Read the model definition and answer for the solid it produces. Units are mm, in the model's axes. Face numbers are marked on the shaded views. A direction names the side the tool comes from. Give positions to 0.01 mm unless a question says otherwise; leave off trailing zeros. Write each loop counter-clockwise with the first axis right and the second up, starting at its lowest first coordinate (ties: lowest second). Pieces come first, ordered by that corner, then holes. Notation, with made-up numbers: (-30.75, 18) - (-22.75, 18) arc R20 cw to (-22.75, 32) - close; hole circle Ø3 at (2, -23.75). An arc over 180 degrees is marked (long way). Answer as CSV lines item,"result".
```python
from build123d import *

# Parameters (mm, degrees)
SKICA1_W                 = 55
SKICA1_H                 = 25
P_IDAT_VYSUNUT_M1_DEPTH  = 5
ODEBRAT_VYSUNUT_M1_DEPTH = 10
SKICA3_W                 = 15
SKICA3_H                 = 25
ODEBRAT_VYSUNUT_M2_DEPTH = 2.5
M4_D_RA_S_V_L_4_DEPTH    = 2.5


# Read off the part's stored shape, not the designer's step: M4 díra s vůlí4
with BuildPart() as part:
    # Skica1 → Přidat vysunutím1 (new body)
    with BuildSketch(Plane.XY):
        Rectangle(SKICA1_W, SKICA1_H)
    extrude(amount=P_IDAT_VYSUNUT_M1_DEPTH)

    # Skica2 → Odebrat vysunutím1 (cut)
    with BuildSketch(Plane.XY.offset(5)):
        with BuildLine():
            Line((-12.5, 3.5), (-8.1, 3.5))
            ThreePointArc((-8.1, 3.5), (-7.936021317, 2.6864759), (-7.469693846, 2))
            Line((-7.469693846, 2), (-4.530306154, 2))
            ThreePointArc((-4.530306154, 2), (-4.063978683, 2.6864759), (-3.9, 3.5))
            Line((-3.9, 3.5), (-2.1, 3.5))
            ThreePointArc((-2.1, 3.5), (-1.936021317, 2.6864759), (-1.469693846, 2))
            Line((-1.469693846, 2), (1.469693846, 2))
            ThreePointArc((1.469693846, 2), (1.936021317, 2.6864759), (2.1, 3.5))
            Line((2.1, 3.5), (3.9, 3.5))
            ThreePointArc((3.9, 3.5), (4.063978683, 2.6864759), (4.530306154, 2))
            Line((4.530306154, 2), (7.469693846, 2))
            ThreePointArc((7.469693846, 2), (7.936021317, 2.6864759), (8.1, 3.5))
            Line((8.1, 3.5), (12.5, 3.5))
            Line((12.5, 3.5), (12.5, 12.5))
            Line((12.5, 12.5), (-12.5, 12.5))
            Line((-12.5, 12.5), (-12.5, 3.5))
        make_face()
    extrude(amount=-ODEBRAT_VYSUNUT_M1_DEPTH, mode=Mode.SUBTRACT)

    # Skica3 → Odebrat vysunutím2 (cut)
    with BuildSketch(Plane.XY.offset(5)):
        with Locations((-20, 0)):
            Rectangle(SKICA3_W, SKICA3_H)
        with Locations((20, 0)):
            Rectangle(SKICA3_W, SKICA3_H)
    extrude(amount=-ODEBRAT_VYSUNUT_M2_DEPTH, mode=Mode.SUBTRACT)

    # M4 díra s vůlí4 outline → M4 díra s vůlí4 (cut)
    with BuildSketch(Plane.XY):
        with BuildLine():
            Line((-20.25, 12.5), (-24.75, 12.5))
            Line((-24.75, 12.5), (-24.75, -7.75))
            ThreePointArc((-24.75, -7.75), (-22.5, -10), (-20.25, -7.75))
            Line((-20.25, -7.75), (-20.25, 12.5))
        make_face()
        with BuildLine():
            Line((24.75, 12.5), (20.25, 12.5))
            Line((20.25, 12.5), (20.25, -7.75))
            ThreePointArc((20.25, -7.75), (22.5, -10), (24.75, -7.75))
            Line((24.75, -7.75), (24.75, 12.5))
        make_face()
    extrude(amount=M4_D_RA_S_V_L_4_DEPTH, mode=Mode.SUBTRACT)


solid = part.part
```
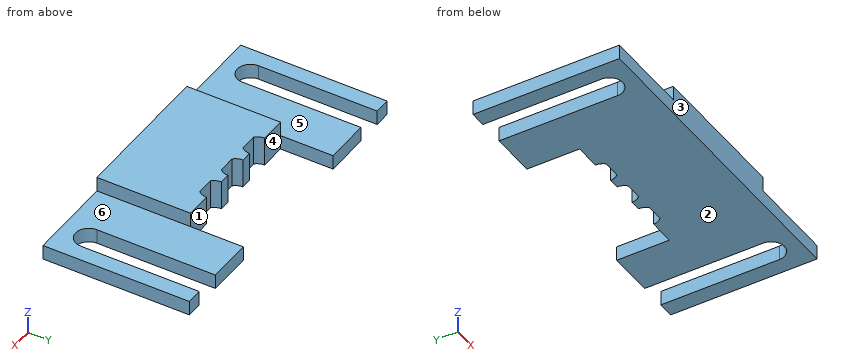
(1) For the marked faces 3, 4, 5 and 6, determine the directions among +Z, -Z, +X, -X, +Y, -Y from which every point of the face is accessible in a straight line to the end or side of a thin tool.
Worked out:
face 3,"+Z, -Z, +X, -X, -Y"
face 4,"+Z, -Z, +Y"
face 5,"+Z, -X, +Y, -Y"
face 6,"+Z, +X, +Y, -Y"
(2) Find the intervals of material crossed by L1, parallel to X at y = -4.5, z = 1.1; L2, parallel to X at y = 9, z = 2; L3, parallel to X at y = 3.25, z = 4.05, in increasing order.
Worked out:
L1,"x = -27.5 to -24.75, -20.25 to 20.25, 24.75 to 27.5"
L2,"x = -27.5 to -24.75, -20.25 to -12.5, 12.5 to 20.25, 24.75 to 27.5"
L3,"x = -12.5 to -8.09, -3.91 to -2.09, 2.09 to 3.91, 8.09 to 12.5"
(3) A cutting plane is placed at B-B (z = 3.2). Write down the section's boundary in (x, y), and give its area (3 significant figures).
Worked out:
outline,"(-12.5, -12.5) - (12.5, -12.5) - (12.5, 3.5) - (8.1, 3.5) arc R2.1 cw to (7.47, 2) - (4.53, 2) arc R2.1 cw to (3.9, 3.5) - (2.1, 3.5) arc R2.1 cw to (1.47, 2) - (-1.47, 2) arc R2.1 cw to (-2.1, 3.5) - (-3.9, 3.5) arc R2.1 cw to (-4.53, 2) - (-7.47, 2) arc R2.1 cw to (-8.1, 3.5) - (-12.5, 3.5) - close"
area,"383 mm^2"
(4) The mould has two halves that part along X. Classify the marked faces 1 and 2: +X half, -X half, draft (parallel to the pull), parting line (faces both ways), or undercut.
Worked out:
face 1,"undercut"
face 2,"draft"
(5) A cutting plane is placed at C-C (x = -18). Write down the section's boundary in (y, z).
Worked out:
outline,"(-12.5, 0) - (12.5, 0) - (12.5, 2.5) - (-12.5, 2.5) - close"
(6) A cutting plane is placed at D-D (x = 22). Write down the section's boundary in (y, z), and give its area (3 significant figures).
Worked out:
outline,"(-12.5, 0) - (-9.94, 0) - (-9.94, 2.5) - (-12.5, 2.5) - close"
area,"6.39 mm^2"
(7) Each of these flat-tipped pins is pushed along its axis until it touches: P1, Ø1.5, axis at x = -6, z = 3, coming from the +Y side; P2, Ø2, axis at x = 2.5, z = 3, coming from the +Y side; P3, Ø1.2, axis at y = -7.5, z = 4, coming from the -X side. Where does it stop, or does it pass through?
Worked out:
P1,"stops at y = 2"
P2,"stops at y = 3.5"
P3,"stops at x = -12.5"
(8) A cutting plane is placed at A-A (y = -2.5). Write down the section's boundary in (x, z), and give its area (4 significant figures).
Worked out:
outline,"(-27.5, 0) - (-24.75, 0) - (-24.75, 2.5) - (-27.5, 2.5) - close; (-20.25, 0) - (20.25, 0) - (20.25, 2.5) - (12.5, 2.5) - (12.5, 5) - (-12.5, 5) - (-12.5, 2.5) - (-20.25, 2.5) - close; (24.75, 0) - (27.5, 0) - (27.5, 2.5) - (24.75, 2.5) - close"
area,"177.5 mm^2"
